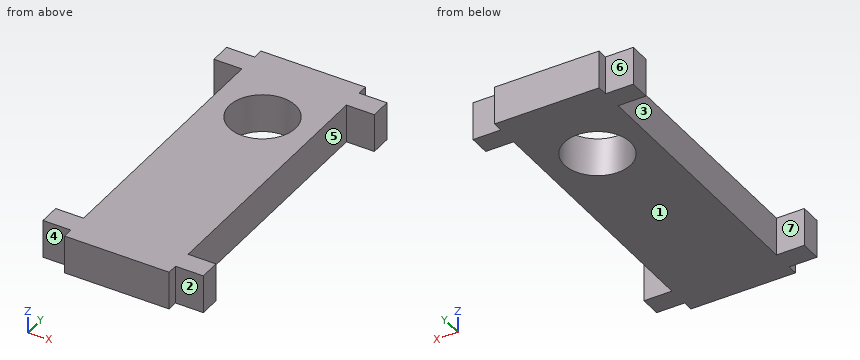
from build123d import *

# Parameters (mm, degrees)
ESQUISSE1_R        = 9.5
BOSS_EXTRU_1_DEPTH = 11


with BuildPart() as part:
    # Esquisse1 → Boss.-Extru.1 (new body)
    with BuildSketch(Plane.XY):
        Polygon((0, 81), (0, 6), (-8, 6), (-8, 0), (0, 0), (0, -3), (30, -3), (30, 0), (38, 0), (38, 6), (30, 6), (30, 81), (38, 81), (38, 87), (30, 87), (30, 90), (25, 90), (5, 90), (0, 90), (0, 87), (-8, 87), (-8, 81), align=None)
        with Locations((15, 66)):
            Circle(ESQUISSE1_R, mode=Mode.SUBTRACT)
    extrude(amount=BOSS_EXTRU_1_DEPTH)


solid = part.part
Check sheet for the modelled part. Datum: model origin and axes. Units: mm. Face numbers are marked on the shaded views. A direction names the side the tool comes from. Round coordinates to 2 decimals unless told otherwise and drop trailing zeros. Loops run counter-clockwise (first coordinate to the right, second up) from the corner with the lowest first, then second, coordinate; pieces in that order, holes last. Notation, with made-up numbers: (-21.75, 59) -> (14.25, 59) arc R25 cw to (14.25, 82) -> close; hole circle Ø11 at (36.5, 89.5). An arc over 180 degrees is marked (long way). Put each result on its own line as item: value. Start each with the question number.
1. Access from +Z, -Z, +X, -X, +Y, -Y to the whole of each face (thin tool, end or side, straight path). Record for the marked faces 4, 5, 6 and 7.
2. Section check A-A (z = 7.5). Enter the section's corners in (x, y), plus the area to 3 significant figures.
3. Scan lines: probe 1 along Y at (x, z) = (-5, 1.25); probe 2 along Y at (x, z) = (15, 8.25); probe 3 along X at (y, z) = (48, 2). Record each from-to range of solid material in increasing order.
4. Gauge pin test, flat ends, axial feed: pin 1 (3 mm diameter, centred on y = 62, z = 5, fed in from -X); pin 2 (2.5 mm diameter, centred on x = 34, z = 5, fed in from +Y); pin 3 (4 mm diameter, centred on x = 33.5, z = 6, fed in from -Y). Record the tip position at first contact, or that the pin passes through.
5. Draft check along Y on the marked faces 1, 2 and 3. Enter one of: +Y half, -Y half, draft (parallel to the pull), parting line (faces both ways), or undercut.
6. Section check D-D (y = 38). Enter the section's corners in (x, z).
7. Section check C-C (y = 66). Enter the section's corners in (x, z), plus the area to 3 significant figures.
8. Section check B-B (x = 15). Enter the section's corners in (y, z), plus the area to 3 significant figures.
Findings:
1. face 4: +Z, -Z, -X, -Y
1. face 5: +Z, -Z, +X
1. face 6: +Z, -Z, -X, +Y
1. face 7: +Z, -Z, -X
2. outline: (-8, 0) -> (0, 0) -> (0, -3) -> (30, -3) -> (30, 0) -> (38, 0) -> (38, 6) -> (30, 6) -> (30, 81) -> (38, 81) -> (38, 87) -> (30, 87) -> (30, 90) -> (0, 90) -> (0, 87) -> (-8, 87) -> (-8, 81) -> (0, 81) -> (0, 6) -> (-8, 6) -> close; hole circle Ø19 at (15, 66)
2. area: 2,700 mm^2
3. probe 1: y = 0 to 6, 81 to 87
3. probe 2: y = -3 to 56.5, 75.5 to 90
3. probe 3: x = 0 to 30
4. pin 1: stops at x = 0
4. pin 2: stops at y = 87
4. pin 3: stops at y = 0
5. face 1: draft
5. face 2: -Y half
5. face 3: undercut
6. outline: (0, 0) -> (30, 0) -> (30, 11) -> (0, 11) -> close
7. outline: (0, 0) -> (5.5, 0) -> (5.5, 11) -> (0, 11) -> close; (24.5, 0) -> (30, 0) -> (30, 11) -> (24.5, 11) -> close
7. area: 121 mm^2
8. outline: (-3, 0) -> (56.5, 0) -> (56.5, 11) -> (-3, 11) -> close; (75.5, 0) -> (90, 0) -> (90, 11) -> (75.5, 11) -> close
8. area: 814 mm^2
